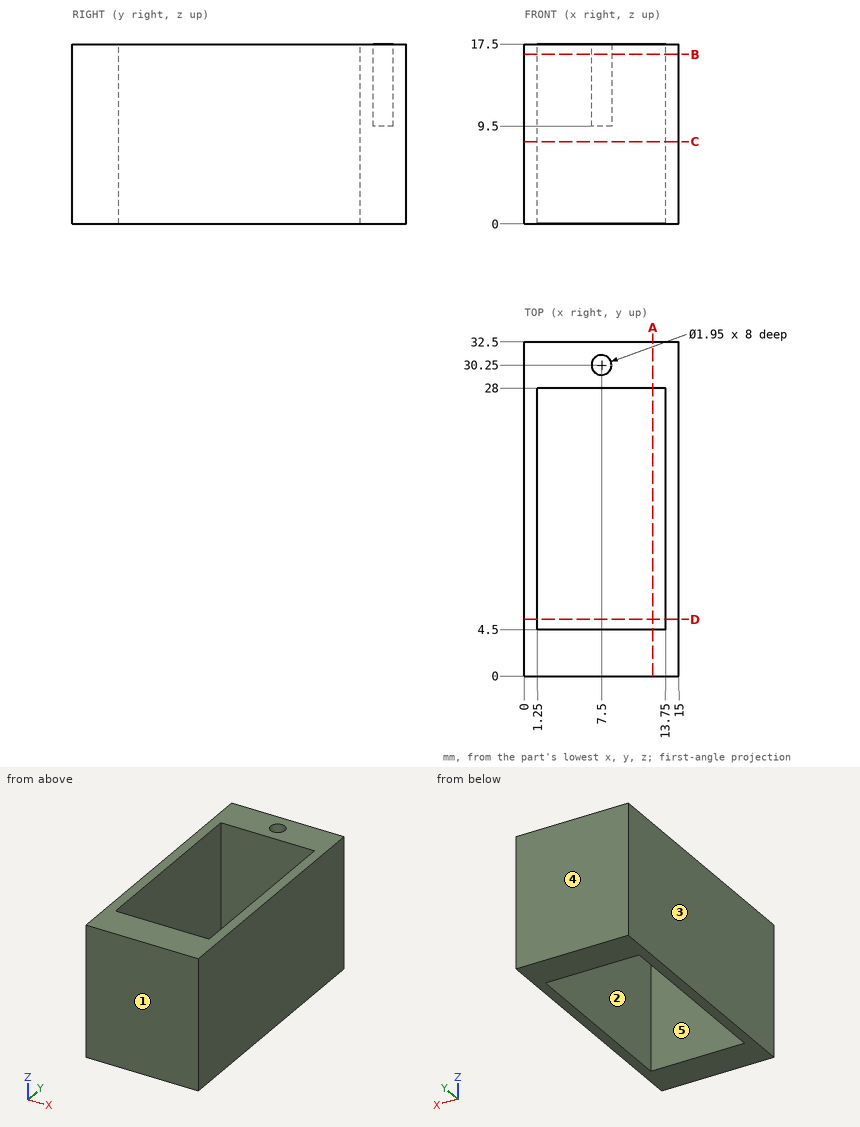
Can you work these out from the drawing? Everything is in mm from the part's minimum corner. A direction names the side the tool comes from. Give positions to 0.01 mm unless a question says otherwise; leave off trailing zeros. Loops run counter-clockwise (first coordinate to the right, second up) from the corner with the lowest first, then second, coordinate; pieces in that order, holes last. Notation, with made-up numbers: (-14, -39) -> (42, -39) arc R21 ccw to (42, -33) -> close; hole circle Ø9 at (26.5, 3). An arc over 180 degrees is marked (long way). Put each result on its own line as item: value.
(1) Imagine slicing it at A-A on x = 12.5. Write out the boundary of the cut face in (y, z).
Computed:
outline: (0, 0) -> (4.5, 0) -> (4.5, 17.5) -> (0, 17.5) -> close; (28, 0) -> (32.5, 0) -> (32.5, 17.5) -> (28, 17.5) -> close
(2) For the marked faces 1 and 2, which set-ups out of +Z, -Z, +X, -X, +Y, -Y let a thin tool reach every point of the face, with its end or its side?
Computed:
face 1: +Z, -Z, +X, -X, -Y
face 2: +Z, -Z
(3) Please list where these lines run through material, in increasing order: probe 1 along Y at (x, z) = (7.5, 13) (3 decimals); probe 2 along Y at (x, z) = (10.25, 5); probe 3 along X at (y, z) = (26, 9.25). Write a range as [from, to].
Computed:
probe 1: [0, 4.5], [28, 29.275], [31.225, 32.5]
probe 2: [0, 4.5], [28, 32.5]
probe 3: [0, 1.25], [13.75, 15]
(4) Thinking about a two-plate mould opening in X: for the marked faces 3, 4 and 5, which applies, pulls with the +X half, pulls with the -X half, needs draft (parallel to the pull), parting line crosses it, or undercut?
Computed:
face 3: pulls with the -X half
face 4: needs draft
face 5: undercut
(5) Imagine slicing it at B-B on z = 16.5. Write out the boundary of the cut face in (x, y) (3 decimals), plus the area to 3 significant figures.
Computed:
outline: (0, 0) -> (15, 0) -> (15, 32.5) -> (0, 32.5) -> close; hole (1.25, 4.5) -> (13.75, 4.5) -> (13.75, 28) -> (1.25, 28) -> close; hole circle Ø1.95 at (7.5, 30.25)
area: 191 mm^2
(6) Imagine slicing it at D-D on y = 5.5. Write out the boundary of the cut face in (x, z), plus the area to 4 significant figures.
Computed:
outline: (0, 0) -> (1.25, 0) -> (1.25, 17.5) -> (0, 17.5) -> close; (13.75, 0) -> (15, 0) -> (15, 17.5) -> (13.75, 17.5) -> close
area: 43.75 mm^2
(7) Imagine slicing it at C-C on z = 8. Write out the boundary of the cut face in (x, y).
Computed:
outline: (0, 0) -> (15, 0) -> (15, 32.5) -> (0, 32.5) -> close; hole (1.25, 4.5) -> (13.75, 4.5) -> (13.75, 28) -> (1.25, 28) -> close
